Autodesk Inventor part; units mm, degrees
ref_plane "YZ Plane" through (0, 0, 0) normal (1, 0, 0) x (0, 1, 0)
ref_plane "XZ Plane" through (0, 0, 0) normal (0, 1, 0) x (-1, 0, 0)
ref_plane "XY Plane" through (0, 0, 0) normal (0, 0, 1) x (1, 0, 0)
sketch "Sketch1" plane through (0, 0, 0) normal (0, 0, 1) x (1, 0, 0)
  line L0 (0, 0) -> (3.81, 0)
  line L1 (3.81, 0) -> (3.81, 9.0424)
  line L2 (3.81, 9.0424) -> (0, 9.0424)
  line L3 (0, 9.0424) -> (0, 0)
  dimension "d0" = 3.81
  dimension "d1" = 9.0424
extrude "Extrusion1" add sketch "Sketch1" against normal blind 10.16
sketch "Sketch2" plane through (0, 0, 0) normal (0, 0, 1) x (1, 0, 0)
  line L0 (0.4347, 8.4539) -> (3.4337, 8.4539)
  line L1 (3.4337, 8.4539) -> (3.4337, 0.4129)
  line L2 (3.4337, 0.4129) -> (0.4347, 0.4129)
  line L3 (0.4347, 0.4129) -> (0.4347, 8.4539)
  point P0 (0, 0)
extrude "Extrusion2" cut sketch "Sketch2" against normal blind 10.16
properties part number "IR PART"
Check sheet for the modelled part. Datum: model origin and axes. Units: mm. A direction names the side the tool comes from. Coordinates: 2 decimals unless noted, no trailing zeros. Order: outer loops, then holes, each group sorted by start corner. A loop starts at its lowest first (then second) coordinate and runs counter-clockwise, first axis right, second up. Notation, with made-up numbers: M 10,-17 L 61,-17 A25 cw 61,-5 Z; hole C 73,70 d8. An arc over 180 degrees is marked long. Write each question's results on one line, items separated by ' | '. Start each with the question number.
1. Access from +Z, -Z, +X, -X, +Y, -Y to the whole of each face (thin tool, end or side, straight path). Record for faces 1 (the face through (0.2, 5.2, -10.16)), 2 (the face through (2, 8.454, -5)).
2. Cross-section at B-B on x = 0.8. Record the cut outline in (y, z), and give its area (3 significant figures).
3. Cross-section at C-C on z = -3.5. Record the cut outline in (x, y), and give its area (3 significant figures).
4. Material ranges on probe 1 along Y at (x, z) = (2.3, -1.25); probe 2 along X at (y, z) = (2.5, -8.5), recorded low to high.
5. Mould release check, pull along Y, two halves, no side actions. Record for faces 3 (the face through (2, 0, -5)), 4 (the face through (2, 0.413, -5)), 5 (the face through (0.2, 5.2, 0)): +Y half, -Y half, draft (parallel to the pull), parting line (faces both ways), or undercut.
6. Cross-section at A-A on y = 3.5. Record the cut outline in (x, z).
Checks:
1) face 1: -Z, +X, -X, +Y, -Y | face 2: +Z, -Z
2) outline: M 0,-10.16 L 0.41,-10.16 L 0.41,0 L 0,0 Z; M 8.45,-10.16 L 9.04,-10.16 L 9.04,0 L 8.45,0 Z | area: 10.2 mm²
3) outline: M 0,0 L 3.81,0 L 3.81,9.04 L 0,9.04 Z; hole M 0.43,0.41 L 3.43,0.41 L 3.43,8.45 L 0.43,8.45 Z | area: 10.3 mm²
4) probe 1: y = 0 to 0.41, 8.45 to 9.04 | probe 2: x = 0 to 0.43, 3.43 to 3.81
5) face 3: -Y half | face 4: undercut | face 5: draft
6) outline: M 0,-10.16 L 0.43,-10.16 L 0.43,0 L 0,0 Z; M 3.43,-10.16 L 3.81,-10.16 L 3.81,0 L 3.43,0 Z
